```python
from build123d import *

# Parameters (mm, degrees)
F0_W     = 38.1
F0_H     = 12.7
F1_DEPTH = 6.35
F2_W     = 38.1
F2_H     = 12.7
F3_DEPTH = 38.1
F4_W     = 38.1
F4_H     = 12.7
F4_R     = 3.175
F5_DEPTH = 12.7


with BuildPart() as f1:
    # F0 (on Top) → F1 (new body)
    with BuildSketch(Plane.XY):
        with Locations((3.2120794058, 1.0928753239)):
            Rectangle(F0_W, F0_H)
    extrude(amount=F1_DEPTH)

    # F2 (on face) → F3 (join)
    with BuildSketch(Plane.XY.offset(6.35)):
        with Locations((3.2120794058, 1.0928753239)):
            Rectangle(F2_W, F2_H)
    extrude(amount=F3_DEPTH)

    # F4 (on face) → F5 (cut)
    with BuildSketch(Plane(origin=(0, 0, 0), x_dir=(1, 0, 0), z_dir=(0, 0, -1))):
        with Locations((3.2120794058, -1.0928753239)):
            Rectangle(F4_W, F4_H)
        with Locations((-5.9024819942, -1.0928753239)):
            Circle(F4_R, mode=Mode.SUBTRACT)
        with Locations((3.2120794058, -1.0928753239)):
            Circle(F4_R, mode=Mode.SUBTRACT)
        with Locations((12.3266408058, -1.0928753239)):
            Circle(F4_R, mode=Mode.SUBTRACT)
    extrude(amount=-F5_DEPTH, mode=Mode.SUBTRACT)


solid = f1.part
```
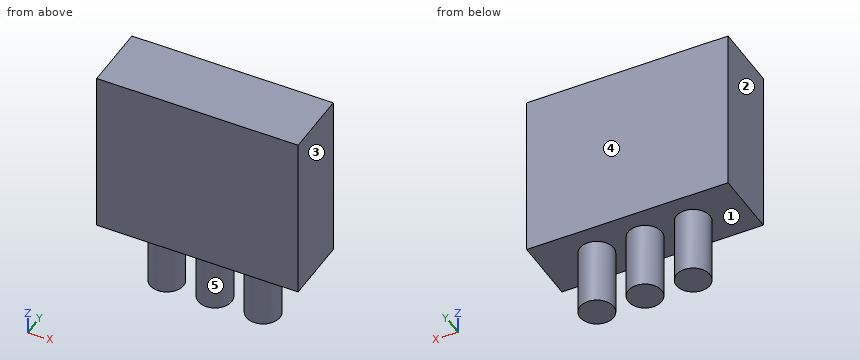
Geometry check sheet. Reference: the model listing, model coordinates, mm. Face numbers are marked on the shaded views. A direction names the side the tool comes from. Give positions to 0.01 mm unless a question says otherwise; leave off trailing zeros. Order: outer loops, then holes, each group sorted by start corner. A loop starts at its lowest first (then second) coordinate and runs counter-clockwise, first axis right, second up.
1. Section check A-A, the plane x = -7.5. Enter the section's corners in (y, z), and give its area (3 significant figures).
2. Release check for a two-part mould opening along X. For the marked faces 1, 2 and 3 record: pulls with the +X half, pulls with the -X half, needs draft (parallel to the pull), parting line crosses it, or undercut.
3. Access from +Z, -Z, +X, -X, +Y, -Y to the whole of each face (thin tool, end or side, straight path). Record for the marked faces 4 and 5.
4. Thickness scan on L1, parallel to X at y = 4, z = 2; L2, parallel to Z at x = 12, y = 6.25; L3, parallel to Y at x = 6, z = 7.5. Record the ranges inside material, lowest first.
5. Section check D-D, the plane x = 14.5. Enter the section's corners in (y, z).
6. Section check C-C, the plane z = 4. Enter the section's corners in (x, y) (3 decimals).
7. Gauge pin test, flat end, axial feed: pin 1 Ø3 at (y, z) = (0.5, 7.5) entering from -X. Record the tip position at first contact, or that the pin passes through.
8. Section check B-B, the plane y = -1. Enter the section's corners in (x, z).
Values follow:
1. outline: (-5.26, 12.7) - (-1.65, 12.7) - (-1.65, 0) - (3.84, 0) - (3.84, 12.7) - (7.44, 12.7) - (7.44, 44.45) - (-5.26, 44.45) - close
1. area: 473 mm2
2. face 1: undercut
2. face 2: pulls with the -X half
2. face 3: pulls with the +X half
3. face 4: +Z, -Z, +X, -X, +Y
3. face 5: -Z
4. L1: x = -7.18 to -4.63, 1.94 to 4.49, 11.05 to 13.6
4. L2: z = 12.7 to 44.45
4. L3: y = -0.43 to 2.61
5. outline: (-5.26, 12.7) - (-1.22, 12.7) - (-1.22, 0) - (3.41, 0) - (3.41, 12.7) - (7.44, 12.7) - (7.44, 44.45) - (-5.26, 44.45) - close
6. outline: circle Ø6.35 at (-5.902, 1.093); circle Ø6.35 at (3.212, 1.093); circle Ø6.35 at (12.327, 1.093)
7. pin 1: stops at x = -9.08
8. outline: (-15.84, 12.7) - (-8.29, 12.7) - (-8.29, 0) - (-3.51, 0) - (-3.51, 12.7) - (0.82, 12.7) - (0.82, 0) - (5.6, 0) - (5.6, 12.7) - (9.94, 12.7) - (9.94, 0) - (14.71, 0) - (14.71, 12.7) - (22.26, 12.7) - (22.26, 44.45) - (-15.84, 44.45) - close
